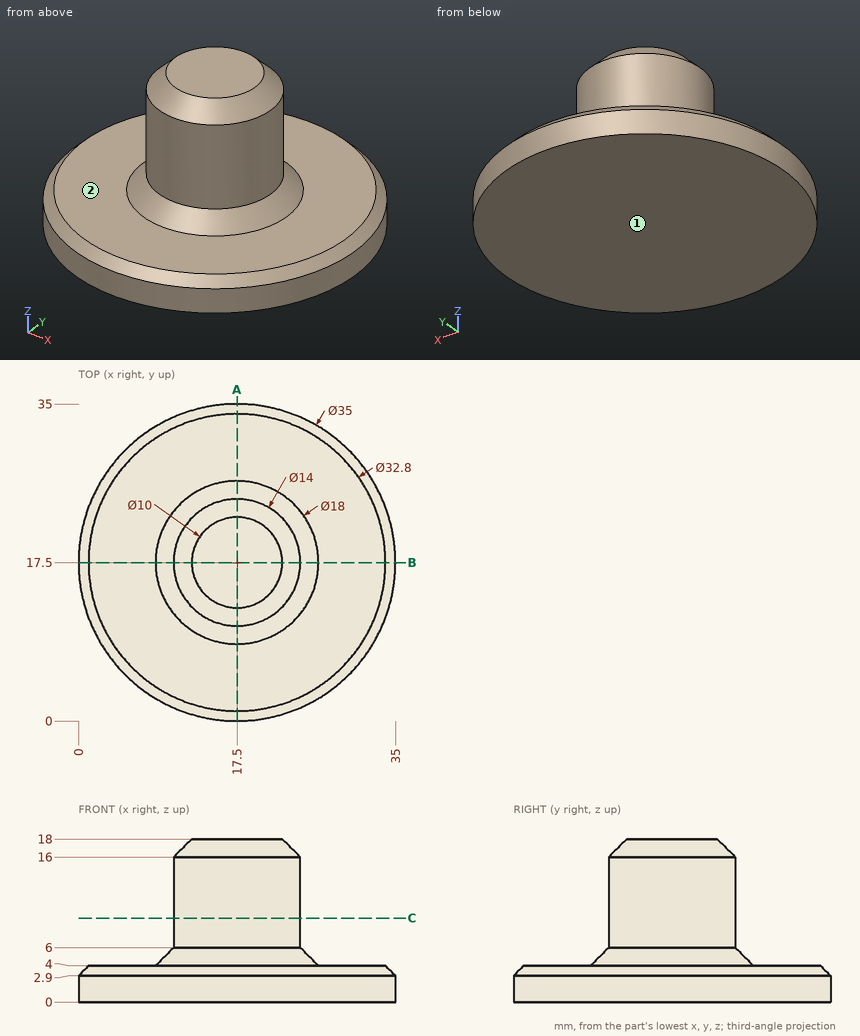
Input: dimensioned drawing with shaded views. Units: mm. Origin: part minimum x, y, z. A direction names the side the tool comes from. Round coordinates to 2 decimals unless told otherwise and drop trailing zeros. Order: outer loops, then holes, each group sorted by start corner. A loop starts at its lowest first (then second) coordinate and runs counter-clockwise, first axis right, second up.
1. Pin query (flat end, axial travel): P1, Ø3, axis at y = 14, z = 2, coming from the -X side; P2, Ø8, axis at x = 6.5, y = 28, coming from the +Z side; P3, Ø3, axis at x = 12, z = 10, coming from the -Y side; P4, Ø8, axis at x = 30, y = 18, coming from the -Z side. Return the tip coordinate at first contact, or that it passes through.
The answers:
P1: stops at x = 0.11
P2: stops at z = 4
P3: stops at y = 11.76
P4: stops at z = 0
2. Cut plane C-C, the plane z = 9.25. Output: boundary loops of the cut face in (x, y).
The answers:
outline: circle Ø14 at (17.5, 17.5)
3. Material intervals for line 1 (Z direction, x = 13.5, y = 6.5); line 2 (X direction, y = 27, z = 1.75); line 3 (X direction, y = 13.5, z = 14), sorted ascending.
The answers:
line 1: z = 0 to 4
line 2: x = 2.8 to 32.2
line 3: x = 11.76 to 23.24
4. Cut plane A-A, the plane x = 17.5. Output: boundary loops of the cut face in (y, z), then the cut area to 3 significant figures.
The answers:
outline: (0, 0) - (35, 0) - (35, 2.9) - (33.9, 4) - (26.5, 4) - (24.5, 6) - (24.5, 16) - (22.5, 18) - (12.5, 18) - (10.5, 16) - (10.5, 6) - (8.5, 4) - (1.1, 4) - (0, 2.9) - close
area: 335 mm2
5. Set-up query: the marked faces 1 and 2. Return all of +Z, -Z, +X, -X, +Y, -Y with unobstructed straight access to the full face (end or side cutting, diameter ignored); none if empty.
The answers:
face 1: -Z, +X, -X, +Y, -Y
face 2: +Z
